Check sheet for the modelled part. Datum: model origin and axes. Units: mm. Give positions to 0.01 mm unless a question says otherwise; leave off trailing zeros. Write each loop counter-clockwise with the first axis right and the second up, starting at its lowest first coordinate (ties: lowest second). Pieces come first, ordered by that corner, then holes. Notation, with made-up numbers: (29.5, -19.5) -> (50.5, -19.5) arc R36 cw to (50.5, 16.5) -> close; hole circle Ø6 at (81, 34). An arc over 180 degrees is marked (long way). Use a Markdown table: item, result. Add a question column.
1. Cross-section at A-A (x = -362). Enter the section's corners in (y, z), then the cut area to 3 significant figures.
2. Cross-section at C-C (z = 1). Count the separate pieces of the cut face and the enclosed holes in it, then the cut area to 3 significant figures.
3. Cross-section at B-B (y = 104). Enter the section's corners in (x, z) (3 decimals), then the cut area to 3 significant figures.
4. Scan lines: probe 1 along X at (y, z) = (361.95, 4) (3 decimals); probe 2 along Y at (x, z) = (-158.75, 3); probe 3 along X at (y, z) = (-342.9, 2) (3 decimals). Record each from-to range of solid material in increasing order. Write a range as [from, to].
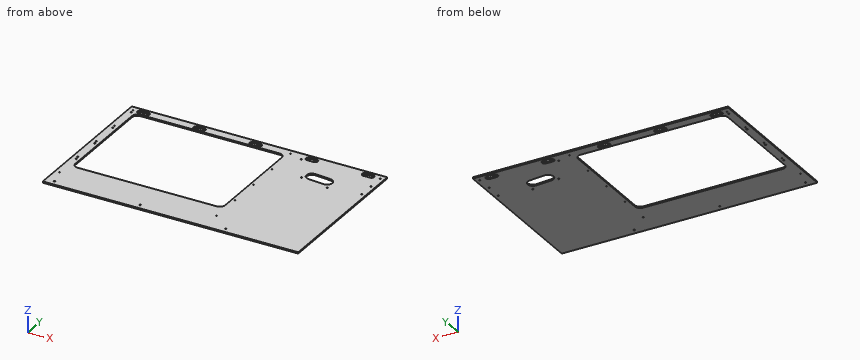
from build123d import *

# Parameters (mm, degrees)
SKETCH1_W                   = 1212.85
SKETCH1_H                   = 736.6
BOSS_EXTRUDE1_DEPTH         = 6.35
H_0_266_DIAMETER_HOLE1_D    = 6.7564
SKETCH2_R                   = 2.45745
SKETCH2_W                   = 711.2
SKETCH2_H                   = 519.684
CUT_EXTRUDE1_DEPTH          = 7.35
H_0_266_DIAMETER_HOLE2_D    = 6.7564
H_0_266_DIAMETER_HOLE3_D    = 6.7564
SKETCH12_R                  = 3.175
CUT_EXTRUDE4_DEPTH          = 7.35
LPATTERN1_COUNT             = 5
LPATTERN1_PITCH             = 266.7
FILLET1_R                   = 3.175
CUT_EXTRUDE5_DEPTH          = 7.35
F_1_4_0_25_DIAMETER_HOLE1_D = 6.35
FILLET2_R                   = 25.4


with BuildPart() as part:
    # Sketch1 → Boss-Extrude1 (new body)
    with BuildSketch(Plane.XY):
        Rectangle(SKETCH1_W, SKETCH1_H)
    extrude(amount=BOSS_EXTRUDE1_DEPTH)

    # H (0.266) Diameter Hole1 (through all)
    with Locations(Plane.XY.offset(6.35)):
        with Locations((-565.15, -342.9), (-158.75, -342.9), (247.65, -342.9)):
            Hole(H_0_266_DIAMETER_HOLE1_D / 2)

    # Sketch2 → Cut-Extrude1 (cut, through all)
    with BuildSketch(Plane.XY.offset(6.35)):
        with Locations((-585.7875, 342.9)):
            Circle(SKETCH2_R)
        with Locations((-585.7875, 190.5)):
            Circle(SKETCH2_R)
        with Locations((-585.7875, 38.1)):
            Circle(SKETCH2_R)
        with Locations((-585.7875, -114.3)):
            Circle(SKETCH2_R)
        with Locations((-585.7875, -266.7)):
            Circle(SKETCH2_R)
        with Locations((160.9725, -266.7)):
            Circle(SKETCH2_R)
        with Locations((160.9725, -114.3)):
            Circle(SKETCH2_R)
        with Locations((160.9725, 38.1)):
            Circle(SKETCH2_R)
        with Locations((160.9725, 190.5)):
            Circle(SKETCH2_R)
        with Locations((160.9725, 342.9)):
            Circle(SKETCH2_R)
        with Locations((-209.55, 64.008)):
            Rectangle(SKETCH2_W, SKETCH2_H)
    extrude(amount=-CUT_EXTRUDE1_DEPTH, mode=Mode.SUBTRACT)

    # H (0.266) Diameter Hole2 (through all)
    with Locations(Plane.XY.offset(6.35)):
        with Locations((-582.6125, 323.596), (-582.6125, 171.196), (-582.6125, 18.796), (-582.6125, -133.604)):
            Hole(H_0_266_DIAMETER_HOLE2_D / 2)

    # H (0.266) Diameter Hole3 (through all)
    with Locations(Plane.XY.offset(6.35)):
        with Locations((223.770763786, 324.305909426), (436.157707656, 167.711380391), (301.059784222, 190.437399182)):
            Hole(H_0_266_DIAMETER_HOLE3_D / 2)

    # Sketch12 → Cut-Extrude4 (cut, through all)
    with BuildSketch(Plane.XY.offset(6.35)):
        with Locations((-536.575, 361.95)):
            Circle(SKETCH12_R)
        with BuildLine():
            Line((-552.45, 355.6), (-520.7, 355.6))
            ThreePointArc((-520.7, 355.6), (-508, 342.9), (-520.7, 330.2))
            Line((-520.7, 330.2), (-552.45, 330.2))
            ThreePointArc((-552.45, 330.2), (-565.15, 342.9), (-552.45, 355.6))
        make_face()
    cut_extrude4 = extrude(amount=-CUT_EXTRUDE4_DEPTH, mode=Mode.SUBTRACT)

    # LPattern1: Cut-Extrude4 ×5
    with Locations(*[(i * LPATTERN1_PITCH, 0, 0) for i in range(1, LPATTERN1_COUNT)]):
        add(cut_extrude4, mode=Mode.SUBTRACT)

    # Fillet1
    fillet1_edges = [part.edges().sort_by_distance(p)[0] for p in [
        (606.425, -368.3, 3.175),
        (-606.425, -368.3, 3.175),
        (-606.425, 368.3, 3.175),
        (606.425, 368.3, 3.175),
    ]]
    fillet(fillet1_edges, radius=FILLET1_R)

    # Sketch14 → Cut-Extrude5 (cut, through all)
    with BuildSketch(Plane.XY.offset(6.35)):
        with BuildLine():
            Line((336.240912114, 244.52397913), (412.150948109, 237.882711533))
            ThreePointArc((412.150948109, 237.882711533), (435.240537575, 210.365610336), (407.723436378, 187.27602087))
            Line((407.723436378, 187.27602087), (331.813400383, 193.917288467))
            ThreePointArc((331.813400383, 193.917288467), (308.723810917, 221.434389664), (336.240912114, 244.52397913))
        make_face()
    extrude(amount=-CUT_EXTRUDE5_DEPTH, mode=Mode.SUBTRACT)

    # 1/4 (0.25) Diameter Hole1 (through all)
    with Locations(Plane.XY.offset(6.35)):
        with Locations((587.375, 342.9), (587.375, 266.7), (587.375, 190.5)):
            Hole(F_1_4_0_25_DIAMETER_HOLE1_D / 2)

    # Fillet2
    fillet2_edges = [part.edges().sort_by_distance(p)[0] for p in [
        (-565.15, -195.834, 3.175),
        (-565.15, 323.85, 3.175),
        (146.05, 323.85, 3.175),
        (146.05, -195.834, 3.175),
    ]]
    fillet(fillet2_edges, radius=FILLET2_R)


solid = part.part
Worked answers:
| question | item | result |
|---|---|---|
| 1 | outline | (-368.3, 0) -> (-195.83, 0) -> (-195.83, 6.35) -> (-368.3, 6.35) -> close; (323.85, 0) -> (368.3, 0) -> (368.3, 6.35) -> (323.85, 6.35) -> close |
| 1 | area | 1,380 mm² |
| 2 | separate pieces | 1 |
| 2 | enclosed holes | 35 |
| 2 | area | 511,000 mm² |
| 3 | outline | (-606.425, 0) -> (-565.15, 0) -> (-565.15, 6.35) -> (-606.425, 6.35) -> close; (146.05, 0) -> (606.425, 0) -> (606.425, 6.35) -> (146.05, 6.35) -> close |
| 3 | area | 3,190 mm² |
| 4 | probe 1 | x = [-606.425, -539.75], [-533.4, -273.05], [-266.7, -6.35], [0, 260.35], [266.7, 527.05], [533.4, 606.425] |
| 4 | probe 2 | y = [-368.3, -346.28], [-339.52, -195.83], [323.85, 368.3] |
| 4 | probe 3 | x = [-606.425, -568.528], [-561.772, -162.128], [-155.372, 244.272], [251.028, 606.425] |
